from build123d import *

# Parameters (mm, degrees)
F1_DEPTH = 63.5
F2_DEPTH = 25.4
F3_DEPTH = 7.9375
F0_W     = 45.5656475117
F0_H     = 19.05
F5_R     = 6.35


with BuildPart() as f1:
    # F0 (on Front) → F1 (new body, symmetric)
    with BuildSketch(Plane.XZ):
        Polygon((22.225, 9.525), (-41.275, 9.525), (-41.275, -9.525), (41.275, -9.525), (41.275, 9.525), align=None)
    extrude(amount=F1_DEPTH, both=True)

    # F0 (on Front) → F2 (join, symmetric)
    with BuildSketch(Plane.XZ):
        with BuildLine():
            Line((22.225, 27.0002), (22.225, 9.525))
            Line((22.225, 9.525), (41.275, 9.525))
            Line((41.275, 9.525), (41.275, 27.0002))
            ThreePointArc((41.275, 27.0002), (45.9246798487, 38.2255201513), (57.15, 42.8752))
            Line((57.15, 42.8752), (60.325, 42.8752))
            Line((60.325, 42.8752), (60.325, 61.9252))
            Line((60.325, 61.9252), (57.15, 61.9252))
            ThreePointArc((57.15, 61.9252), (32.4542956671, 51.6959043329), (22.225, 27.0002))
        make_face()
    extrude(amount=F2_DEPTH, both=True)

    # F0 (on Front) → F3 (join, symmetric)
    with BuildSketch(Plane.XZ):
        with BuildLine():
            add(Edge.make_bspline(
                [(-41.275, 9.525), (-38.2011030893, 43.7511456965), (22.4494743774, 75.5444682119), (57.15, 61.9252)],
                knots=[0, 0, 0, 0, 111.5045361635, 111.5045361635, 111.5045361635, 111.5045361635], degree=3))
            Line((-41.275, 9.525), (22.225, 9.525))
            Line((22.225, 9.525), (22.225, 27.0002))
            ThreePointArc((22.225, 27.0002), (32.4542956671, 51.6959043329), (57.15, 61.9252))
        make_face()
    extrude(amount=F3_DEPTH, both=True)

    # F0 (on Front) → F4 (revolve)
    with BuildSketch(Plane.XZ):
        with Locations((83.1078237558, 52.4002)):
            Rectangle(F0_W, F0_H)
    revolve(axis=Axis((60.325, 0, 52.3875), (0, 0, 1)))

    # F5
    f5_edges = [f1.edges().sort_by_distance(p)[0] for p in [
        (41.275, -63.5, 0),
        (-41.275, -63.5, 0),
        (41.275, 63.5, 0),
        (-41.275, 63.5, 0),
    ]]
    fillet(f5_edges, radius=F5_R)


solid = f1.part
Verification items for the finished model (mm, model axes). A direction names the side the tool comes from. Coordinates: 2 decimals unless noted, no trailing zeros. Write each loop counter-clockwise with the first axis right and the second up, starting at its lowest first coordinate (ties: lowest second). Pieces come first, ordered by that corner, then holes. Notation, with made-up numbers: M 70.25,57.5 L 76.25,57.5 A27 ccw 76.25,75.5 Z; hole C 28.25,36.5 d9. An arc over 180 degrees is marked long. Use CSV: the item, a comma, the result in double quotes.
Q1. Thickness scan on line 1 along Y through (x, z) = (-12, 27); line 2 along Z through (x, y) = (7.5, -57) (3 decimals); line 3 along Z through (x, y) = (38, -24) (3 decimals). Record the ranges inside material, lowest first. Write a range as [from, to].
Computed values:
line 1,"[-7.94, 7.94]"
line 2,"[-9.525, 9.525]"
line 3,"[-9.525, 61.925]"
Q2. Go/stop test with flat-tipped pins: P1, Ø12, axis at y = -26, z = 16.5, coming from the -X side (3 decimals); P2, Ø11, axis at y = 18, z = 14, coming from the +X side (3 decimals); P3, Ø5, axis at y = 25.5, z = 34.5, coming from the +X side. Record where each tip stops, or that it passes through.
Computed values:
P1,"x = 22.225"
P2,"x = 41.275"
P3,"x = 44.82"
Q3. Section check A-A, the plane z = -2. Enter the section's corners in (x, y) (3 decimals).
Computed values:
outline,"M -41.275,-57.15 A6.35 ccw -34.925,-63.5 L 34.925,-63.5 A6.35 ccw 41.275,-57.15 L 41.275,57.15 A6.35 ccw 34.925,63.5 L -34.925,63.5 A6.35 ccw -41.275,57.15 Z"
Q4. Mould release check, pull along Z, two halves, no side actions. Record for faces 4 (the cylindrical face through (45.8, -0.4, 38.1)), 5 (the flat face through (61, 1, 42.875)), 6 (the cylindrical face through (-39.464, 61.59, -0.133)): pulls with the +Z half, pulls with the -Z half, needs draft (parallel to the pull), parting line crosses it, or undercut.
Computed values:
face 4,"pulls with the -Z half"
face 5,"undercut"
face 6,"needs draft"
Q5. Section check C-C, the plane y = 52. Enter the section's corners in (x, z) (3 decimals).
Computed values:
outline,"M -41.275,-9.525 L 41.275,-9.525 L 41.275,9.525 L -41.275,9.525 Z"
Q6. Section check B-B, the plane y = -30.5. Enter the section's corners in (x, z) (3 decimals).
Computed values:
outline,"M -41.275,-9.525 L 41.275,-9.525 L 41.275,9.525 L -41.275,9.525 Z; M 26.473,42.875 L 94.177,42.875 L 94.177,61.925 L 26.473,61.925 Z"
Q7. Set-up check for faces 1 (the flat face through (32, 25.4, 26)), 2 (the flat face through (37, 7.938, 63)), 3 (the flat face through (22.225, -17, 18)): record each of +Z, -Z, +X, -X, +Y, -Y from which the full face is reachable in a straight line by a thin tool's end or side.
Computed values:
face 1,"+X, -X, +Y"
face 2,"+Z, +X, -X, +Y"
face 3,"-X, -Y"
